from build123d import *

# Parameters (mm, degrees)
SKETCH1_W           = 20
SKETCH1_H           = 5.65
BOSS_EXTRUDE1_DEPTH = 3.175
FILLET1_R           = 2
SKETCH2_R           = 1.52
CUT_EXTRUDE1_DEPTH  = 3.175


with BuildPart() as part:
    # Sketch1 → Boss-Extrude1 (new body)
    with BuildSketch(Plane.XY):
        Rectangle(SKETCH1_W, SKETCH1_H)
    extrude(amount=BOSS_EXTRUDE1_DEPTH)

    # Fillet1
    fillet1_edges = [part.edges().sort_by_distance(p)[0] for p in [
        (10, -2.825, 1.5875),
        (-10, -2.825, 1.5875),
        (-10, 2.825, 1.5875),
        (10, 2.825, 1.5875),
    ]]
    fillet(fillet1_edges, radius=FILLET1_R)

    # Sketch2 → Cut-Extrude1 (cut)
    with BuildSketch(Plane.XY.offset(3.175)):
        with Locations((-7, 0)):
            Circle(SKETCH2_R)
        with Locations((7, 0)):
            Circle(SKETCH2_R)
        with BuildLine():
            Line((-2.525, 1), (2.525, 1))
            ThreePointArc((2.525, 1), (3.525, 0), (2.525, -1))
            Line((2.525, -1), (-2.525, -1))
            ThreePointArc((-2.525, -1), (-3.525, 0), (-2.525, 1))
        make_face()
    extrude(amount=-CUT_EXTRUDE1_DEPTH, mode=Mode.SUBTRACT)


solid = part.part
Source: CAD feature listing. Evaluate the final solid. Frame: model axes, mm. A direction names the side the tool comes from. Give positions to 0.01 mm unless a question says otherwise; leave off trailing zeros. Write each loop counter-clockwise with the first axis right and the second up, starting at its lowest first coordinate (ties: lowest second). Pieces come first, ordered by that corner, then holes. Notation, with made-up numbers: (82.5, 25) -> (98.5, 25) arc R13 ccw to (98.5, 45) -> close; hole circle Ø8 at (83, 37). An arc over 180 degrees is marked (long way). Write item = value, one per line.
Q1. Mould query, pull axis Y, two halves, no side actions, for faces 3 (the face through (0, 1, 2)), 4 (the face through (10, 0, 2)), 5 (the face through (3.525, 0.022, 1.61)), 6 (the face through (-9.43, -2.224, 1.61)). Classes: +Y half, -Y half, draft (parallel to the pull), parting line (faces both ways), or undercut.
Here are the results:
face_3 = undercut
face_4 = draft
face_5 = undercut
face_6 = -Y half
Q2. Cut plane A-A on y = 0. Return loops of the section in (x, z) (3 decimals).
Here are the results:
outline = (-10, 0) -> (-8.52, 0) -> (-8.52, 3.175) -> (-10, 3.175) -> close; (-5.48, 0) -> (-3.525, 0) -> (-3.525, 3.175) -> (-5.48, 3.175) -> close; (3.525, 0) -> (5.48, 0) -> (5.48, 3.175) -> (3.525, 3.175) -> close; (8.52, 0) -> (10, 0) -> (10, 3.175) -> (8.52, 3.175) -> close
Q3. Cut plane B-B on z = 0.5. Return loops of the section in (x, y) (3 decimals).
Here are the results:
outline = (-10, -0.825) arc R2 ccw to (-8, -2.825) -> (8, -2.825) arc R2 ccw to (10, -0.825) -> (10, 0.825) arc R2 ccw to (8, 2.825) -> (-8, 2.825) arc R2 ccw to (-10, 0.825) -> close; hole circle Ø3.04 at (-7, 0); hole (-2.525, -1) -> (2.525, -1) arc R1 ccw to (2.525, 1) -> (-2.525, 1) arc R1 ccw to start; hole circle Ø3.04 at (7, 0)
Q4. Cut plane C-C on x = -1. Return loops of the section in (y, z) (3 decimals), then the cut area to 3 significant figures.
Here are the results:
outline = (-2.825, 0) -> (-1, 0) -> (-1, 3.175) -> (-2.825, 3.175) -> close; (1, 0) -> (2.825, 0) -> (2.825, 3.175) -> (1, 3.175) -> close
area = 11.6 mm²
Q5. Reachability of faces 1 (the face through (0, -1, 2)), 2 (the face through (-0.1, -1.2, 0)) from +Z, -Z, +X, -X, +Y, -Y: full face, straight path, thin tool, end or side. Return the list, or none.
Here are the results:
face_1 = +Z, -Z
face_2 = -Z, +X, -X, +Y, -Y
Q6. Line query: line 1 (Y direction, x = -7, z = 1.65) (3 decimals); line 2 (Y direction, x = -0.5, z = 1.6) (3 decimals); line 3 (X direction, y = -0.55, z = 1.15). Output: solid intervals per line, ascending. Write a range as from..to.
Here are the results:
line_1 = -2.825..-1.52, 1.52..2.825
line_2 = -2.825..-1, 1..2.825
line_3 = -10..-8.42, -5.58..-3.36, 3.36..5.58, 8.42..10
Q7. Cut plane D-D on y = -1.25. Return loops of the section in (x, z) (3 decimals), then the cut area to 3 significant figures.
Here are the results:
outline = (-9.954, 0) -> (-7.865, 0) -> (-7.865, 3.175) -> (-9.954, 3.175) -> close; (-6.135, 0) -> (6.135, 0) -> (6.135, 3.175) -> (-6.135, 3.175) -> close; (7.865, 0) -> (9.954, 0) -> (9.954, 3.175) -> (7.865, 3.175) -> close
area = 52.2 mm²
Q8. First-contact query: pin 1 (1.5 mm diameter, centred on y = -2, z = 1, fed in from -X). Flat tip, straight axial feed; report the tip coordinate or a pass-through.
Here are the results:
pin_1 = -9.95
